Verification items for the finished model (mm, model axes). Face numbers are marked on the shaded views. A direction names the side the tool comes from. Round coordinates to 2 decimals unless told otherwise and drop trailing zeros. Order: outer loops, then holes, each group sorted by start corner. A loop starts at its lowest first (then second) coordinate and runs counter-clockwise, first axis right, second up. Notation, with made-up numbers: M 34.25,2 L 49.25,2 A17 cw 49.25,32 Z; hole C -40,55.5 d8. An arc over 180 degrees is marked long. Use one line per item in the form item = value. Start each with the question number.
Item 1: Cross-section at B-B on y = -114.3. Enter the section's corners in (x, z).
Item 2: Cross-section at C-C on y = 0. Enter the section's corners in (x, z).
Item 3: Go/stop test with flat-tipped pins: pin 1 Ø8 at (y, z) = (-23.5, 4) entering from +X; pin 2 Ø2 at (x, y) = (-64.5, -14) entering from +Z; pin 3 Ø1 at (x, z) = (-15.5, 6.5) entering from -Y; pin 4 Ø10 at (x, z) = (-126, 15) entering from -Y. Record where each tip stops, or that it passes through.
Item 4: Tool access check on the marked faces 5, 6 and 7. Record the directions out of +Z, -Z, +X, -X, +Y, -Y that give a thin tool (end or side, any length) a straight path to the whole face; none if there is none.
Item 5: Cross-section at D-D on y = 28. Enter the section's corners in (x, z), then the cut area to 3 significant figures.
Item 6: Cross-section at A-A on y = 120.65. Enter the section's corners in (x, z), then the cut area to 3 significant figures.
Item 7: Release check for a two-part mould opening along Y. For the marked faces 1, 2, 3 and 4 record: +Y half, -Y half, draft (parallel to the pull), parting line (faces both ways), or undercut.
Item 8: Thickness scan on probe 1 along Z at (x, y) = (-147.75, -114.3); probe 2 along Y at (x, z) = (-46, 19.75) (1 decimal); probe 3 along Y at (x, z) = (-42, 4). Record the ranges inside material, lowest first. Write a range as [from, to].
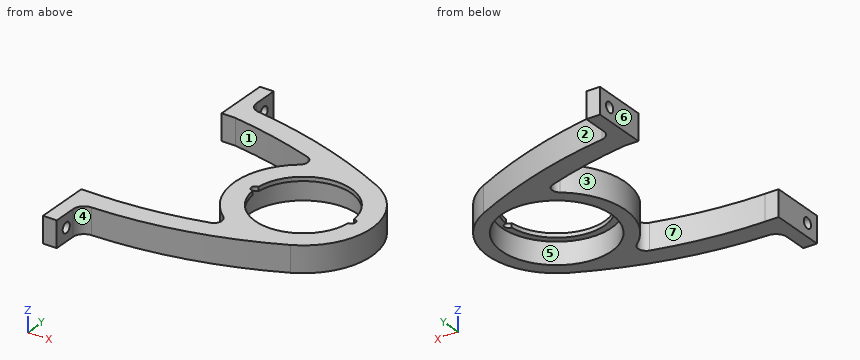
from build123d import *

# Parameters (mm, degrees)
SKETCH1_R           = 50.8
BOSS_EXTRUDE1_DEPTH = 24.13
FILLET1_R           = 10.16
FILLET3_R           = 7.62
SKETCH2_R           = 4.7625
CUT_EXTRUDE1_DEPTH  = 255.906432784
BOSS_EXTRUDE2_START = -3.81
SKETCH3_R           = 50.8
BOSS_EXTRUDE2_DEPTH = 3.81


with BuildPart() as part:
    # Sketch1 → Boss-Extrude1 (new body)
    with BuildSketch(Plane.XY):
        with BuildLine():
            Line((-133.35, 133.35), (-133.35, 82.55))
            Line((-133.35, 82.55), (-120.65, 82.55))
            ThreePointArc((-120.65, 82.55), (-72.294267859, 72.899793875), (-25.200511476, 58.285368844))
            ThreePointArc((-25.200511476, 58.285368844), (-63.5, 0), (-25.200511476, -58.285368844))
            ThreePointArc((-25.200511476, -58.285368844), (-81.753760084, -71.69426344), (-139.7, -76.2))
            Line((-139.7, -76.2), (-152.4, -76.2))
            Line((-152.4, -76.2), (-152.4, -127))
            Line((-152.4, -127), (-139.7, -127))
            Line((-139.7, -127), (-139.7, -95.25))
            ThreePointArc((-139.7, -95.25), (-53.65862904, -85.877953603), (27.94, -57.022858574))
            ThreePointArc((27.94, -57.022858574), (63.5, 0), (27.94, 57.022858574))
            ThreePointArc((27.94, 57.022858574), (-44.521647721, 85.422584161), (-120.65, 101.6))
            Line((-120.65, 101.6), (-120.65, 133.35))
            Line((-120.65, 133.35), (-133.35, 133.35))
        make_face()
        with Locations(Location((0, 0, 0), (0, 0, 180))):
            Circle(SKETCH1_R, mode=Mode.SUBTRACT)
    extrude(amount=BOSS_EXTRUDE1_DEPTH)

    # Fillet1
    fillet1_edges = [part.edges().sort_by_distance(p)[0] for p in [
        (-120.65, 101.6, 12.065),
        (-139.7, -95.25, 12.065),
    ]]
    fillet(fillet1_edges, radius=FILLET1_R)

    # Fillet3
    fillet3_edges = [part.edges().sort_by_distance(p)[0] for p in [
        (-25.200511476, -58.285368844, 12.065),
        (-25.200511476, 58.285368844, 12.065),
    ]]
    fillet(fillet3_edges, radius=FILLET3_R)

    # Sketch2 → Cut-Extrude1 (cut, through all)
    with BuildSketch(Plane.ZY.offset(152.4)):
        with Locations(Location((12.065, -114.3, 0), (0, 0, 270))):
            Circle(SKETCH2_R)
        with Locations(Location((12.065, 120.65, 0), (0, 0, 270))):
            Circle(SKETCH2_R)
    extrude(amount=-CUT_EXTRUDE1_DEPTH, mode=Mode.SUBTRACT)

    # Sketch3 → Boss-Extrude2 (add)
    with BuildSketch(Plane.XY.offset(24.13).offset(BOSS_EXTRUDE2_START)):
        with Locations(Location((0, 0, 0), (0, 0, 180))):
            Circle(SKETCH3_R)
        with BuildLine():
            ThreePointArc((-44.286714286, -3.806499412), (0, -44.45), (44.286714286, -3.806499412))
            ThreePointArc((44.286714286, -3.806499412), (48.26, 0), (44.286714286, 3.806499412))
            ThreePointArc((44.286714286, 3.806499412), (0, 44.45), (-44.286714286, 3.806499412))
            ThreePointArc((-44.286714286, 3.806499412), (-48.26, 0), (-44.286714286, -3.806499412))
        make_face(mode=Mode.SUBTRACT)
    extrude(amount=BOSS_EXTRUDE2_DEPTH)


solid = part.part
Output values:
q1.outline = M -152.4,0 L -139.7,0 L -139.7,7.3 L -152.4,7.3 Z; M -152.4,16.83 L -139.7,16.83 L -139.7,24.13 L -152.4,24.13 Z
q2.outline = M -63.5,0 L -50.8,0 L -50.8,20.32 L -48.26,20.32 L -48.26,24.13 L -63.5,24.13 Z; M 48.26,20.32 L 50.8,20.32 L 50.8,0 L 63.5,0 L 63.5,24.13 L 48.26,24.13 Z
q3.pin_1 = 60.43
q3.pin_2 = through
q3.pin_3 = -75.19
q3.pin_4 = -95.29
q4.face_5 = -Z
q4.face_6 = +Z, -Z, -X, +Y
q4.face_7 = +Z, -Z, -X
q5.outline = M -56.99,0 L -42.39,0 L -42.39,20.32 L -34.52,20.32 L -34.52,24.13 L -56.99,24.13 Z; M 34.52,20.32 L 42.39,20.32 L 42.39,0 L 56.99,0 L 56.99,24.13 L 34.52,24.13 Z
q5.area = 765 mm2
q6.outline = M -133.35,0 L -120.65,0 L -120.65,7.3 L -133.35,7.3 Z; M -133.35,16.83 L -120.65,16.83 L -120.65,24.13 L -133.35,24.13 Z
q6.area = 185 mm2
q7.face_1 = undercut
q7.face_2 = +Y half
q7.face_3 = undercut
q7.face_4 = -Y half
q8.probe_1 = [0, 7.3], [16.83, 24.13]
q8.probe_2 = [-84, -64.3], [-43.8, -21.6], [21.6, 43.8], [65.4, 85.9]
q8.probe_3 = [-83.02, -63.24], [-47.63, -28.58], [28.58, 47.63], [64.12, 84.66]
